The model under review builds one solid part; all positions refer to its coordinate system, in mm. Give positions to 0.01 mm unless a question says otherwise; leave off trailing zeros. Order: outer loops, then holes, each group sorted by start corner. A loop starts at its lowest first (then second) coordinate and runs counter-clockwise, first axis right, second up. Notation, with made-up numbers: (23.5, 29) - (39.5, 29) arc R23 ccw to (39.5, 43) - close; hole circle Ø2 at (78, 42). An arc over 180 degrees is marked (long way). Use CSV: the item, a comma, the result in double quotes.
```python
from build123d import *

# Parameters (mm, degrees)
SKETCH2_R               = 22.5
BOSS_EXTRUDE1_DEPTH     = 3.175
SKETCH3_R               = 3.25755
SKETCH3_R_2             = 2.15
CUT_EXTRUDE1_DEPTH      = 1
CUT_EXTRUDE1_DEPTH_BACK = 7.35
SKETCH4_R               = 2.25
CUT_EXTRUDE2_DEPTH      = 10


with BuildPart() as part:
    # Sketch2 → Boss-Extrude1 (new body, symmetric)
    with BuildSketch(Plane.XY):
        Polygon((-34.925, 0), (34.925, 0), (34.925, 70.1), (34.925, 102.6), (34.925, 117.6), (-34.925, 117.6), (-34.925, 102.6), (-34.925, 70.1), align=None)
        with Locations((0, 70.1)):
            Circle(SKETCH2_R, mode=Mode.SUBTRACT)
    extrude(amount=BOSS_EXTRUDE1_DEPTH, both=True)

    # Sketch3 → Cut-Extrude1 (cut, two sides)
    with BuildSketch(Plane.XY.offset(3.175)) as cut_extrude1_sk:
        with Locations((-25.425, 12.7)):
            Circle(SKETCH3_R)
        with Locations((25.425, 12.7)):
            Circle(SKETCH3_R)
        with Locations((22.425, 111.1)):
            Circle(SKETCH3_R_2)
    extrude(amount=CUT_EXTRUDE1_DEPTH, mode=Mode.SUBTRACT)
    extrude(cut_extrude1_sk.sketch, amount=-CUT_EXTRUDE1_DEPTH_BACK, mode=Mode.SUBTRACT)

    # Sketch4 → Cut-Extrude2 (cut)
    with BuildSketch(Plane.XY.offset(3.175)):
        with Locations((28, 96.1)):
            Circle(SKETCH4_R)
        with Locations((-28, 44.1)):
            Circle(SKETCH4_R)
        with Locations((28, 44.1)):
            Circle(SKETCH4_R)
        with Locations((-28, 96.1)):
            Circle(SKETCH4_R)
    extrude(amount=-CUT_EXTRUDE2_DEPTH, mode=Mode.SUBTRACT)


solid = part.part
```
Item 1: Take a section at B-B, the plane z = -2. State how many separate pieces and enclosed holes the cut face has, and give its area (3 significant figures).
Results list:
separate pieces,"1"
enclosed holes,"8"
area,"6,480 mm2"
Item 2: Take a section at C-C, the plane y = 70.1. Give the boundary of the cut face in (x, z) (3 decimals), and give its area (3 significant figures).
Results list:
outline,"(-34.925, -3.175) - (-22.5, -3.175) - (-22.5, 3.175) - (-34.925, 3.175) - close; (22.5, -3.175) - (34.925, -3.175) - (34.925, 3.175) - (22.5, 3.175) - close"
area,"158 mm2"
Item 3: Take a section at D-D, the plane x = 7. Give the boundary of the cut face in (y, z) (3 decimals).
Results list:
outline,"(0, -3.175) - (48.717, -3.175) - (48.717, 3.175) - (0, 3.175) - close; (91.483, -3.175) - (117.6, -3.175) - (117.6, 3.175) - (91.483, 3.175) - close"
Item 4: Mouldability with a two-part tool opening along X and no side actions: class faces 1 (the face through (28.434, 11.452, 0.044)), 2 (the face through (34.925, 58, 0)), 3 (the face through (0, 117.6, 0)) as pulls with the +X half, pulls with the -X half, needs draft (parallel to the pull), parting line crosses it, or undercut.
Results list:
face 1,"undercut"
face 2,"pulls with the +X half"
face 3,"needs draft"
Item 5: Take a section at A-A, the plane y = 12.7. Give the boundary of the cut face in (x, z) (3 decimals), and give its area (3 significant figures).
Results list:
outline,"(-34.925, -3.175) - (-28.683, -3.175) - (-28.683, 3.175) - (-34.925, 3.175) - close; (-22.167, -3.175) - (22.167, -3.175) - (22.167, 3.175) - (-22.167, 3.175) - close; (28.683, -3.175) - (34.925, -3.175) - (34.925, 3.175) - (28.683, 3.175) - close"
area,"361 mm2"
Item 6: Wall thickness on L1, parallel to Y at x = -25.5, z = 2.5; L2, parallel to Y at x = -28, z = -1.5; L3, parallel to Y at x = -12.5, z = 1: over which ranges is each line inside the solid? List them lowest first.
Results list:
L1,"y = 0 to 9.44, 15.96 to 117.6"
L2,"y = 0 to 10.7, 14.7 to 41.85, 46.35 to 93.85, 98.35 to 117.6"
L3,"y = 0 to 51.39, 88.81 to 117.6"
